CAD build for the part. Positions are in the model's coordinates, mm. Give positions to 0.01 mm unless a question says otherwise; leave off trailing zeros. Write each loop counter-clockwise with the first axis right and the second up, starting at its lowest first coordinate (ties: lowest second). Pieces come first, ordered by that corner, then holes. Notation, with made-up numbers: (5, 36) -> (31, 36) arc R18 cw to (31, 50) -> close; hole circle Ø6 at (68.25, 86). An arc over 180 degrees is marked (long way). Use one line per item in the form item = value. Start each with the question number.
from build123d import *

# Parameters (mm, degrees)
BOSS_EXTRUDE3_DEPTH = 3.2


with BuildPart() as part:
    # Sketch1 → Boss-Extrude3 (new body)
    with BuildSketch(Plane(origin=(0, 0, 0), x_dir=(1, 0, 0), z_dir=(0, 1, 0))):
        Polygon((80.018202502, -34.385003933), (87.688185358, -34.385003933), (87.688185358, -31.185003933), (95.358168214, -31.185003933), (95.358168214, -34.385003933), (103.02815107, -34.385003933), (103.02815107, -31.185003933), (110.698133926, -31.185003933), (110.698133926, -34.385003933), (118.368116782, -34.385003933), (118.368116782, -18.996696241), (124.110679366, -18.996696241), (124.110679366, -6.808388549), (118.368116782, -6.808388549), (118.368116782, 5.379919143), (124.110679366, 5.379919143), (124.110679366, 17.568226836), (118.368116782, 17.568226836), (118.368116782, 29.756534528), (124.110679366, 29.756534528), (124.110679366, 41.94484222), (118.368116782, 41.94484222), (118.368116782, 54.133149913), (124.110679366, 54.133149913), (124.110679366, 66.321457605), (118.368116782, 66.321457605), (118.368116782, 78.509765297), (124.110679366, 78.509765297), (124.110679366, 90.69807299), (118.368116782, 90.69807299), (118.368116782, 102.886380682), (124.110679366, 102.886380682), (124.110679366, 115.074688374), (118.368116782, 115.074688374), (118.368116782, 127.262996067), (74.275639917, 127.262996067), (74.275639917, 115.074688374), (80.018202502, 115.074688374), (80.018202502, 102.886380682), (74.275639917, 102.886380682), (74.275639917, 90.69807299), (80.018202502, 90.69807299), (80.018202502, 78.509765297), (74.275639917, 78.509765297), (74.275639917, 66.321457605), (80.018202502, 66.321457605), (80.018202502, 54.133149913), (74.275639917, 54.133149913), (74.275639917, 41.94484222), (80.018202502, 41.94484222), (80.018202502, 29.756534528), (74.275639917, 29.756534528), (74.275639917, 17.568226836), (80.018202502, 17.568226836), (80.018202502, 5.379919143), (74.275639917, 5.379919143), (74.275639917, -6.808388549), (80.018202502, -6.808388549), (80.018202502, -18.996696241), (74.275639917, -18.996696241), (74.275639917, -31.185003933), (80.018202502, -31.185003933), align=None)
    extrude(amount=BOSS_EXTRUDE3_DEPTH)


solid = part.part
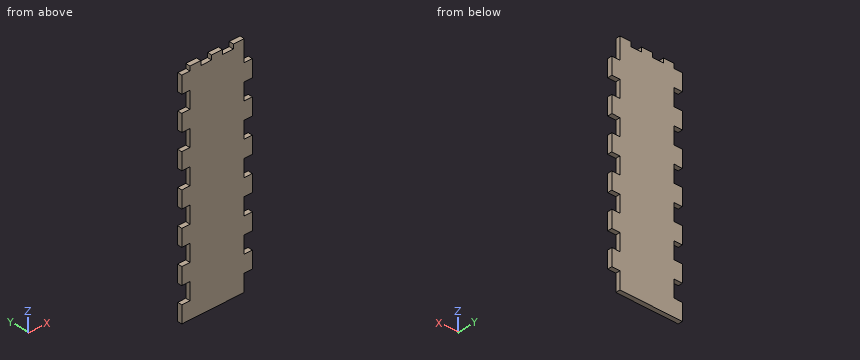
1) Wall check: line 1 along Z through (x, y) = (121, 2.6); line 2 along X through (y, z) = (2.4, -61); line 3 along X through (y, z) = (2.05, -50). Give the ranges that are in metal, low to high. Write a range as from..to.
2) Pin check, flat tips, straight feed: pin 1 (1.6 mm diameter, centred on y = 1.5, z = -21.5, fed in from +X); pin 2 (1.6 mm diameter, centred on x = 120, y = 1.5, fed in from +Z); pin 3 (1.6 mm diameter, centred on y = 2.5, z = -37, fed in from -X). Stop position of each tip, or through.
3) Cut at A-A (x = 92.5). Give the cut face in (y, z) (3 decimals), and give its area (3 significant figures).
4) Cut at B-B (z = -97). Give the cut face in (x, y).
Final values:
q1.line_1 = -115.07..-102.89, -90.7..-78.51, -66.32..-54.13, -41.94..-29.76, -17.57..-5.38, 6.81..19
q1.line_2 = 80.02..124.11
q1.line_3 = 74.28..118.37
q2.pin_1 = 118.37
q2.pin_2 = 19
q2.pin_3 = 80.02
q3.outline = (0, -127.263) -> (3.2, -127.263) -> (3.2, 31.185) -> (0, 31.185) -> close
q3.area = 507 mm^2
q4.outline = (74.28, 0) -> (118.37, 0) -> (118.37, 3.2) -> (74.28, 3.2) -> close
